from build123d import *

# Parameters (mm, degrees)
SKETCH1_W           = 900
SKETCH1_H           = 530
BOSS_EXTRUDE1_DEPTH = 15
SKETCH3_R           = 25
CUT_EXTRUDE1_DEPTH  = 16


with BuildPart() as part:
    # Sketch1 → Boss-Extrude1 (new body)
    with BuildSketch(Plane.XY):
        with Locations((450, 265)):
            Rectangle(SKETCH1_W, SKETCH1_H)
    extrude(amount=BOSS_EXTRUDE1_DEPTH)

    # Sketch3 → Cut-Extrude1 (cut, through all)
    with BuildSketch(Plane(origin=(0, 0, 0), x_dir=(-1, 0, 0), z_dir=(0, 0, -1))):
        with Locations((-780, 150)):
            Circle(SKETCH3_R)
        with Locations((-680, 165)):
            Circle(SKETCH3_R)
        with Locations((-580, 180)):
            Circle(SKETCH3_R)
        with Locations((-480, 195)):
            Circle(SKETCH3_R)
    extrude(amount=-CUT_EXTRUDE1_DEPTH, mode=Mode.SUBTRACT)


solid = part.part
Geometry: final body of the model. Coordinates: model frame, mm. Give positions to 0.01 mm unless a question says otherwise; leave off trailing zeros. Order: outer loops, then holes, each group sorted by start corner. A loop starts at its lowest first (then second) coordinate and runs counter-clockwise, first axis right, second up. Notation, with made-up numbers: (-19, -19) -> (8, -19) arc R29 cw to (8, 7) -> close; hole circle Ø2 at (62, -8.75). An arc over 180 degrees is marked (long way). Answer as a JSON object with one key per item and string values.
Q1. Draft query along X for faces 1 (the flat face through (444, 269, 0)), 2 (the cylindrical face through (556.154, 187.509, 7.395)). Return one class per face: released by +X, released by -X, zero draft, split by the parting line, or undercut.
Entries:
{"face 1": "zero draft", "face 2": "undercut"}
Q2. Section B-B (x = 480). Output: boundary loops of the cut face in (y, z), plus the area to 3 significant figures.
Entries:
{"outline": "(0, 0) -> (170, 0) -> (170, 15) -> (0, 15) -> close; (220, 0) -> (530, 0) -> (530, 15) -> (220, 15) -> close", "area": "7,200 mm^2"}
Q3. Material intervals for probe 1 along Y at (x, z) = (780, 7.5); probe 2 along Y at (x, z) = (680, 11), sorted ascending.
Entries:
{"probe 1": "y = 0 to 125, 175 to 530", "probe 2": "y = 0 to 140, 190 to 530"}
Q4. Section A-A (z = 10). Output: boundary loops of the cut face in (x, y), plus the area to 3 significant figures.
Entries:
{"outline": "(0, 0) -> (900, 0) -> (900, 530) -> (0, 530) -> close; hole circle Ø50 at (480, 195); hole circle Ø50 at (580, 180); hole circle Ø50 at (680, 165); hole circle Ø50 at (780, 150)", "area": "469,000 mm^2"}
